from build123d import *

# Parameters (mm, degrees)
SKETCH1_R          = 582.5
SKETCH1_R_2        = 552.5
BASE_FLANGE1_DEPTH = 2.5
SKETCH8_R          = 5
CUT_EXTRUDE1_DEPTH = 10


# Read off the part's stored shape, not the designer's step: Edge-Flange1
# Sheet-metal steps are written as plain solids
with BuildPart() as part:
    # Sketch1 → Base-Flange1 (new body)
    with BuildSketch(Plane(origin=(0, 0, 0), x_dir=(1, 0, 0), z_dir=(0, 1, 0))):
        with Locations(Location((0, 0, 0), (0, 0, 270))):
            Circle(SKETCH1_R)
        with Locations(Location((0, 0, 0), (0, 0, 270))):
            Circle(SKETCH1_R_2, mode=Mode.SUBTRACT)
    extrude(amount=-BASE_FLANGE1_DEPTH)

    # Edge-Flange1 outline → Edge-Flange1 (revolve, cut)
    with BuildSketch(Plane.XY):
        with BuildLine():
            Line((552.5, -2.5), (552.645898034, -2.5))
            ThreePointArc((552.645898034, -2.5), (553.908349934, -0.69375696), (556, 0))
            Line((556, 0), (552.5, 0))
            Line((552.5, 0), (552.5, -2.5))
        make_face()
    revolve(axis=Axis((0, 0, 0), (0, 1, 0)), mode=Mode.SUBTRACT)

    # Edge-Flange1 2 outline → Edge-Flange1 2 (revolve)
    with BuildSketch(Plane.XY):
        with BuildLine():
            Line((552.5, -3.5), (552.5, -33.5))
            Line((552.5, -33.5), (555, -33.5))
            Line((555, -33.5), (555, -3.5))
            ThreePointArc((555, -3.5), (555.292893219, -2.792893219), (556, -2.5))
            Line((556, -2.5), (552.645898034, -2.5))
            ThreePointArc((552.645898034, -2.5), (552.536666571, -2.994706462), (552.5, -3.5))
        make_face()
    revolve(axis=Axis((0, 0, 0), (0, 1, 0)))

    # Sketch8 → Cut-Extrude1 (cut)
    with BuildSketch(Plane(origin=(0, 0, 0), x_dir=(1, 0, 0), z_dir=(0, 1, 0))):
        with Locations(Location((175.367144308, 539.724572998, 0), (0, 0, 270))):
            Circle(SKETCH8_R)
        with Locations(Location((333.568130676, 459.117144308, 0), (0, 0, 270))):
            Circle(SKETCH8_R)
        with Locations(Location((0, 567.5, 0), (0, 0, 270))):
            Circle(SKETCH8_R)
        with Locations(Location((459.117144308, 333.568130676, 0), (0, 0, 270))):
            Circle(SKETCH8_R)
        with Locations(Location((539.724572998, 175.367144308, 0), (0, 0, 270))):
            Circle(SKETCH8_R)
        with Locations(Location((567.5, 0, 0), (0, 0, 270))):
            Circle(SKETCH8_R)
        with Locations(Location((539.724572998, -175.367144308, 0), (0, 0, 270))):
            Circle(SKETCH8_R)
        with Locations(Location((459.117144308, -333.568130676, 0), (0, 0, 270))):
            Circle(SKETCH8_R)
        with Locations(Location((333.568130676, -459.117144308, 0), (0, 0, 270))):
            Circle(SKETCH8_R)
        with Locations(Location((175.367144308, -539.724572997, 0), (0, 0, 270))):
            Circle(SKETCH8_R)
        with Locations(Location((0, -567.5, 0), (0, 0, 270))):
            Circle(SKETCH8_R)
        with Locations(Location((-175.367144308, -539.724572998, 0), (0, 0, 270))):
            Circle(SKETCH8_R)
        with Locations(Location((-333.568130676, -459.117144308, 0), (0, 0, 270))):
            Circle(SKETCH8_R)
        with Locations(Location((-459.117144308, -333.568130676, 0), (0, 0, 270))):
            Circle(SKETCH8_R)
        with Locations(Location((-539.724572997, -175.367144308, 0), (0, 0, 270))):
            Circle(SKETCH8_R)
        with Locations(Location((-567.5, 0, 0), (0, 0, 270))):
            Circle(SKETCH8_R)
        with Locations(Location((-539.724572997, 175.367144308, 0), (0, 0, 270))):
            Circle(SKETCH8_R)
        with Locations(Location((-459.117144308, 333.568130676, 0), (0, 0, 270))):
            Circle(SKETCH8_R)
        with Locations(Location((-333.568130676, 459.117144308, 0), (0, 0, 270))):
            Circle(SKETCH8_R)
        with Locations(Location((-175.367144308, 539.724572997, 0), (0, 0, 270))):
            Circle(SKETCH8_R)
    extrude(amount=-CUT_EXTRUDE1_DEPTH, mode=Mode.SUBTRACT)


solid = part.part
The model under review builds one solid part; all positions refer to its coordinate system, in mm. A direction names the side the tool comes from. Round coordinates to 2 decimals unless told otherwise and drop trailing zeros. Write each loop counter-clockwise with the first axis right and the second up, starting at its lowest first coordinate (ties: lowest second). Pieces come first, ordered by that corner, then holes. Notation, with made-up numbers: M 20,-22 L 68,-22 A24 cw 68,-8 Z; hole C -29.5,53.25 d3. An arc over 180 degrees is marked long. Use a Markdown table: item, result. Add a question column.
Q1. Machinability: for faces 4 (the face through (-299, 0, 472)), 5 (the face through (-72.25, -18.29, -550.277)), which of the approach directions +Z, -Z, +X, -X, +Y, -Y give a long, thin tool a straight path to every point of the face, cutting with its end or side? Answer none if there is none.
Q2. To check wall thickness, follow line 1 (Z direction, x = 0, y = -21.75); line 2 (Y direction, x = 208, z = 527); line 3 (X direction, y = -26, z = -41). State the ranges of each line that lie inside material, in increasing order.
Q3. The part is to be moulded in two halves that separate along Z. For faces 1 (the face through (-354.442, -1.232, -462.252)), 2 (the face through (-299, -2.5, 472)), 3 (the face through (526.987, -18.71, -165.956)), say which applies: pulls with the +Z half, pulls with the -Z half, needs draft (parallel to the pull), parting line crosses it, or undercut.
Q4. Insertion check: pin 1 (9 mm diameter, centred on x = 0, z = 567.5, fed in from -Y); pin 2 (1.5 mm diameter, centred on x = -41, y = -27.5, fed in from -Z); pin 3 (8 mm diameter, centred on y = -19.5, z = -2, fed in from +X); pin 4 (12 mm diameter, centred on x = -296, y = -16, fed in from +Z). Each pin has a flat end and moves straight along its axis. Give the tip position at first contact, or say it passes through.
Q5. We need section A-A, the plane y = -15. State the section outline as (x, z) points, plus the area to 3 significant figures.
Findings below:
| question | item | result |
|---|---|---|
| 1 | face 4 | +Z, -Z, +X, -X, +Y |
| 1 | face 5 | -Y |
| 2 | line 1 | z = -555 to -552.5, 552.5 to 555 |
| 2 | line 2 | y = -2.5 to 0 |
| 2 | line 3 | x = -553.48 to -550.98, 550.98 to 553.48 |
| 3 | face 1 | parting line crosses it |
| 3 | face 2 | needs draft |
| 3 | face 3 | undercut |
| 4 | pin 1 | passes through |
| 4 | pin 2 | stops at z = -553.54 |
| 4 | pin 3 | stops at x = 555 |
| 4 | pin 4 | stops at z = 473.21 |
| 5 | outline | C 0,0 d1110; hole C 0,0 d1105 |
| 5 | area | 8,700 mm² |
